Here's how the part is built. I have some questions about the finished solid (model axes, mm). Coordinates: 2 decimals unless noted, no trailing zeros. Order: outer loops, then holes, each group sorted by start corner. A loop starts at its lowest first (then second) coordinate and runs counter-clockwise, first axis right, second up. Notation, with made-up numbers: (85.5, 67.25) - (93.5, 67.25) arc R22 ccw to (93.5, 91.25) - close; hole circle Ø2 at (88, -33). An arc over 180 degrees is marked (long way). Answer in a Markdown table with one row per item. Add a question column.
Item 1: I want a section at B-B (y = -25.5). Please give me the cut outline in (x, z).
Item 2: I want a section at D-D (z = 0.65). Count the separate pieces of the cut face and the enclosed holes in it, plus the area to 3 significant figures.
Item 3: I want a section at A-A (y = 6.5). Please give me the cut outline in (x, z).
Item 4: I want a section at C-C (x = -40.2). Please give me the cut outline in (y, z), plus the area to 3 significant figures.
Item 5: If I drill on line 1 along X through (y, z) = (5, 0.5); line 2 along Y through (x, z) = (-40.2, 0.5); line 3 along X through (y, z) = (11.5, 0.5), over which ranges is the centre line in solid material (lowest first)? Write a range as from..to.
Item 6: Will these pins go through, and if not, where does the flat tip stop? pin 1 Ø4 at (x, y) = (-40.2, -25.5) entering from -Z; pin 2 Ø0.8 at (x, z) = (2, 0.5) entering from -Y.
```python
from build123d import *

# Parameters (mm, degrees)
BOSS_EXTRUDE1_DEPTH = 1.5
SKETCH2_R           = 2.5
CUT_EXTRUDE1_DEPTH  = 56.936928768


with BuildPart() as part:
    # Sketch1 → Boss-Extrude1 (new body)
    with BuildSketch(Plane.XY):
        with BuildLine():
            Line((-36.25, -13), (-36.25, 13))
            ThreePointArc((-36.25, 13), (-39.308359466, 17.14885926), (-43.325461287, 20.378331156))
            ThreePointArc((-43.325461287, 20.378331156), (-44.549693467, 29.632815837), (-35.244739735, 28.883104448))
            ThreePointArc((-35.244739735, 28.883104448), (-32.441546823, 25.602755414), (-29, 23))
            Line((-29, 23), (29, 23))
            ThreePointArc((29, 23), (32.441546823, 25.602755414), (35.244739735, 28.883104448))
            ThreePointArc((35.244739735, 28.883104448), (44.549693467, 29.632815837), (43.325461287, 20.378331156))
            ThreePointArc((43.325461287, 20.378331156), (39.308359466, 17.14885926), (36.25, 13))
            Line((36.25, 13), (36.25, -13))
            ThreePointArc((36.25, -13), (39.308359466, -17.14885926), (43.325461287, -20.378331156))
            ThreePointArc((43.325461287, -20.378331156), (44.549693467, -29.632815837), (35.244739735, -28.883104448))
            ThreePointArc((35.244739735, -28.883104448), (32.441546823, -25.602755414), (29, -23))
            Line((29, -23), (-29, -23))
            ThreePointArc((-29, -23), (-32.441546823, -25.602755414), (-35.244739735, -28.883104448))
            ThreePointArc((-35.244739735, -28.883104448), (-44.549693467, -29.632815837), (-43.325461287, -20.378331156))
            ThreePointArc((-43.325461287, -20.378331156), (-39.308359466, -17.14885926), (-36.25, -13))
        make_face()
    extrude(amount=BOSS_EXTRUDE1_DEPTH)

    # Sketch2 → Cut-Extrude1 (cut, through all)
    with BuildSketch(Plane.XY.offset(1.5)):
        with Locations((-40.2, 25.5)):
            Circle(SKETCH2_R)
        with Locations(Location((-40.2, -25.5, 0), (0, 0, 180))):
            Circle(SKETCH2_R)
        with Locations((40.2, -25.5)):
            Circle(SKETCH2_R)
        with Locations(Location((40.2, 25.5, 0), (0, 0, 180))):
            Circle(SKETCH2_R)
        with BuildLine():
            Line((-22.396410464, 19.85), (-12.826410464, 19.85))
            ThreePointArc((-12.826410464, 19.85), (-11.949193754, 19.33009462), (-11.984116418, 18.310981689))
            Line((-11.984116418, 18.310981689), (-15.482345258, 12.844493329))
            ThreePointArc((-15.482345258, 12.844493329), (-16.190773525, 12.392512169), (-16.993732126, 12.640332796))
            Line((-16.993732126, 12.640332796), (-23.065503286, 18.106821155))
            ThreePointArc((-23.065503286, 18.106821155), (-23.33, 19.208344217), (-22.396410464, 19.85))
        make_face()
        with BuildLine():
            Line((-29.733467607, 11.735), (-29.733467607, -11.735))
            ThreePointArc((-29.733467607, -11.735), (-29.226272987, -12.605139562), (-28.219181892, -12.592618915))
            Line((-28.219181892, -12.592618915), (-25.217515688, -10.792618915))
            ThreePointArc((-25.217515688, -10.792618915), (-24.861661841, -10.42780538), (-24.731801403, -9.935))
            Line((-24.731801403, -9.935), (-24.731801403, 9.935))
            ThreePointArc((-24.731801403, 9.935), (-24.861661841, 10.42780538), (-25.217515688, 10.792618915))
            Line((-25.217515688, 10.792618915), (-28.219181892, 12.592618915))
            ThreePointArc((-28.219181892, 12.592618915), (-29.226272987, 12.605139562), (-29.733467607, 11.735))
        make_face()
        with BuildLine():
            Line((-2.396410464, 19.85), (2.403589536, 19.85))
            ThreePointArc((2.403589536, 19.85), (2.918821443, 19.707050805), (3.286749377, 19.319072165))
            Line((3.286749377, 19.319072165), (6.471749377, 13.322416847))
            ThreePointArc((6.471749377, 13.322416847), (6.445640341, 12.338112776), (5.588589536, 11.853344682))
            Line((5.588589536, 11.853344682), (-5.581410464, 11.853344682))
            ThreePointArc((-5.581410464, 11.853344682), (-6.438461269, 12.338112776), (-6.464570304, 13.322416847))
            Line((-6.464570304, 13.322416847), (-3.279570304, 19.319072165))
            ThreePointArc((-3.279570304, 19.319072165), (-2.91164237, 19.707050805), (-2.396410464, 19.85))
        make_face()
        with BuildLine():
            Line((22.403589536, 20.151728768), (12.833589536, 20.151728768))
            ThreePointArc((12.833589536, 20.151728768), (11.956372827, 19.631823388), (11.99129549, 18.612710457))
            Line((11.99129549, 18.612710457), (15.48952433, 13.146222097))
            ThreePointArc((15.48952433, 13.146222097), (16.197952597, 12.694240937), (17.000911199, 12.942061564))
            Line((17.000911199, 12.942061564), (23.072682359, 18.408549924))
            ThreePointArc((23.072682359, 18.408549924), (23.337179073, 19.510072985), (22.403589536, 20.151728768))
        make_face()
        with BuildLine():
            Line((17.000911199, -12.942061564), (23.072682359, -18.408549924))
            ThreePointArc((23.072682359, -18.408549924), (23.337179073, -19.510072985), (22.403589536, -20.151728768))
            Line((22.403589536, -20.151728768), (12.833589536, -20.151728768))
            ThreePointArc((12.833589536, -20.151728768), (11.956372827, -19.631823388), (11.99129549, -18.612710457))
            Line((11.99129549, -18.612710457), (15.48952433, -13.146222097))
            ThreePointArc((15.48952433, -13.146222097), (16.197952597, -12.694240937), (17.000911199, -12.942061564))
        make_face()
        with BuildLine():
            Line((-6.464570304, -13.322416847), (-3.279570304, -19.319072165))
            ThreePointArc((-3.279570304, -19.319072165), (-2.91164237, -19.707050805), (-2.396410464, -19.85))
            Line((-2.396410464, -19.85), (2.403589536, -19.85))
            ThreePointArc((2.403589536, -19.85), (2.918821443, -19.707050805), (3.286749377, -19.319072165))
            Line((3.286749377, -19.319072165), (6.471749377, -13.322416847))
            ThreePointArc((6.471749377, -13.322416847), (6.445640341, -12.338112776), (5.588589536, -11.853344682))
            Line((5.588589536, -11.853344682), (-5.581410464, -11.853344682))
            ThreePointArc((-5.581410464, -11.853344682), (-6.438461269, -12.338112776), (-6.464570304, -13.322416847))
        make_face()
        with BuildLine():
            Line((-16.993732126, -12.640332796), (-23.065503286, -18.106821155))
            ThreePointArc((-23.065503286, -18.106821155), (-23.33, -19.208344217), (-22.396410464, -19.85))
            Line((-22.396410464, -19.85), (-12.826410464, -19.85))
            ThreePointArc((-12.826410464, -19.85), (-11.949193754, -19.33009462), (-11.984116418, -18.310981689))
            Line((-11.984116418, -18.310981689), (-15.482345258, -12.844493329))
            ThreePointArc((-15.482345258, -12.844493329), (-16.190773525, -12.392512169), (-16.993732126, -12.640332796))
        make_face()
        with BuildLine():
            Line((25.217515688, 10.792618915), (28.219181892, 12.592618915))
            ThreePointArc((28.219181892, 12.592618915), (29.226272987, 12.605139562), (29.733467607, 11.735))
            Line((29.733467607, 11.735), (29.733467607, -11.735))
            ThreePointArc((29.733467607, -11.735), (29.226272987, -12.605139562), (28.219181892, -12.592618915))
            Line((28.219181892, -12.592618915), (25.217515688, -10.792618915))
            ThreePointArc((25.217515688, -10.792618915), (24.861661841, -10.42780538), (24.731801403, -9.935))
            Line((24.731801403, -9.935), (24.731801403, 9.935))
            ThreePointArc((24.731801403, 9.935), (24.861661841, 10.42780538), (25.217515688, 10.792618915))
        make_face()
    extrude(amount=-CUT_EXTRUDE1_DEPTH, mode=Mode.SUBTRACT)


solid = part.part
```
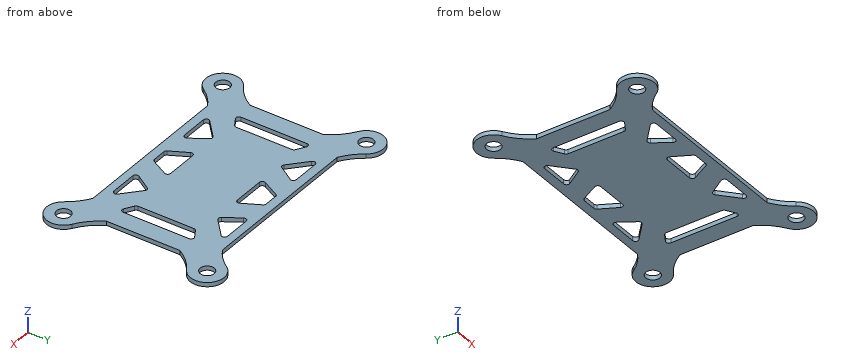
Values follow:
| question | item | result |
|---|---|---|
| 1 | outline | (-46.2, 0) - (-42.7, 0) - (-42.7, 1.5) - (-46.2, 1.5) - close; (-37.7, 0) - (-32.33, 0) - (-32.33, 1.5) - (-37.7, 1.5) - close; (32.33, 0) - (37.7, 0) - (37.7, 1.5) - (32.33, 1.5) - close; (42.7, 0) - (46.2, 0) - (46.2, 1.5) - (42.7, 1.5) - close |
| 2 | separate pieces | 1 |
| 2 | enclosed holes | 12 |
| 2 | area | 3,210 mm^2 |
| 3 | outline | (-36.25, 0) - (-29.73, 0) - (-29.73, 1.5) - (-36.25, 1.5) - close; (-24.73, 0) - (24.73, 0) - (24.73, 1.5) - (-24.73, 1.5) - close; (29.73, 0) - (36.25, 0) - (36.25, 1.5) - (29.73, 1.5) - close |
| 4 | outline | (-31.5, 0) - (-28, 0) - (-28, 1.5) - (-31.5, 1.5) - close; (-23, 0) - (-18.02, 0) - (-18.02, 1.5) - (-23, 1.5) - close; (18.02, 0) - (23, 0) - (23, 1.5) - (18.02, 1.5) - close; (28, 0) - (31.5, 0) - (31.5, 1.5) - (28, 1.5) - close |
| 4 | area | 25.4 mm^2 |
| 5 | line 1 | x = -36.25..-29.73, -24.73..24.73, 29.73..36.25 |
| 5 | line 2 | y = -31.5..-28, -23..-18.02, 18.02..23, 28..31.5 |
| 5 | line 3 | x = -36.25..-29.73, -26.4..26.4, 29.73..36.25 |
| 6 | pin 1 | passes through |
| 6 | pin 2 | stops at y = -23 |
